Input: part model. Units: mm. Frame: model coordinates. A direction names the side the tool comes from. Give positions to 0.01 mm unless a question says otherwise; leave off trailing zeros. Loops run counter-clockwise (first coordinate to the right, second up) from the corner with the lowest first, then second, coordinate; pieces in that order, holes last. Notation, with made-up numbers: (54, -26.5) - (79, -26.5) arc R12 ccw to (79, -12.5) - close; hole circle Ø9 at (54.5, -18.5). An arc over 180 degrees is marked (long way). One line per item, written item: value.
from build123d import *

# Parameters (mm, degrees)
BOSS_EXTRUDE1_DEPTH = 12.7
SKETCH2_R           = 2.413
CUT_EXTRUDE1_DEPTH  = 55.064572735


with BuildPart() as part:
    # Sketch1 → Boss-Extrude1 (new body)
    with BuildSketch(Plane.XY):
        Polygon((0, 0), (0, 38.1), (1.905, 38.1), (1.905, 1.905), (38.1, 1.905), (38.1, 0), align=None)
    extrude(amount=BOSS_EXTRUDE1_DEPTH)

    # Sketch2 → Cut-Extrude1 (cut, through all)
    with BuildSketch(Plane(origin=(1.905, 0, 0), x_dir=(0, 0, -1), z_dir=(1, 0, 0))):
        with Locations(Location((-6.35, 30.734, 0), (0, 0, 90))):
            Circle(SKETCH2_R)
        with Locations(Location((-6.35, 12.954, 0), (0, 0, 90))):
            Circle(SKETCH2_R)
    cut_extrude1 = extrude(amount=-CUT_EXTRUDE1_DEPTH, mode=Mode.SUBTRACT)

    # Mirror1: Cut-Extrude1 across plane
    add(cut_extrude1.mirror(Plane(origin=(0, 0, 0), x_dir=(0, 0, 1), z_dir=(-0.7071067811865471, 0.7071067811865479, 0))), mode=Mode.SUBTRACT)


solid = part.part
Item 1: Draft query along X for faces 1 (the face through (38.1, 1, 6)), 2 (the face through (33.036, 0.966, 7.075)), 3 (the face through (1, 38.1, 6)). Return one class per face: pulls with the +X half, pulls with the -X half, needs draft (parallel to the pull), parting line crosses it, or undercut.
Verdict:
face 1: pulls with the +X half
face 2: undercut
face 3: needs draft
Item 2: Section B-B, the plane x = 29.5. Output: boundary loops of the cut face in (y, z) (3 decimals).
Verdict:
outline: (0, 0) - (1.905, 0) - (1.905, 4.276) - (0, 4.276) - close; (0, 8.424) - (1.905, 8.424) - (1.905, 12.7) - (0, 12.7) - close
Item 3: Access query for faces 4 (the face through (11, 1, 0)), 5 (the face through (1.905, 20, 6)). Directions: +Z, -Z, +X, -X, +Y, -Y. A direction counts if a zero-diameter tool reaches every point of the face in a straight line with its end or side. Return the directions, or none.
Verdict:
face 4: -Z, +X, -X, +Y, -Y
face 5: +Z, -Z, +X, +Y
Item 4: Section C-C, the plane y = 30.5. Output: boundary loops of the cut face in (x, z) (3 decimals), and give its area (3 significant figures).
Verdict:
outline: (0, 0) - (1.905, 0) - (1.905, 3.948) - (0, 3.948) - close; (0, 8.752) - (1.905, 8.752) - (1.905, 12.7) - (0, 12.7) - close
area: 15.0 mm^2
Item 5: Section D-D, the plane z = 10.25. Output: boundary loops of the cut face in (x, y) (3 decimals), and give its area (3 significant figures).
Verdict:
outline: (0, 0) - (38.1, 0) - (38.1, 1.905) - (1.905, 1.905) - (1.905, 38.1) - (0, 38.1) - close
area: 142 mm^2
Item 6: Section A-A, the plane z = 6.35. Output: boundary loops of the cut face in (x, y) (3 decimals).
Verdict:
outline: (0, 0) - (10.541, 0) - (10.541, 1.905) - (1.905, 1.905) - (1.905, 10.541) - (0, 10.541) - close; (0, 15.367) - (1.905, 15.367) - (1.905, 28.321) - (0, 28.321) - close; (0, 33.147) - (1.905, 33.147) - (1.905, 38.1) - (0, 38.1) - close; (15.367, 0) - (28.321, 0) - (28.321, 1.905) - (15.367, 1.905) - close; (33.147, 0) - (38.1, 0) - (38.1, 1.905) - (33.147, 1.905) - close
Item 7: Pin query (flat end, axial travel): P1, Ø6.5, axis at x = 12.954, z = 6.35, coming from the +Y side (3 decimals); P2, Ø5, axis at y = 27, z = 10.5, coming from the +X side (3 decimals). Return the tip coordinate at first contact, or that it passes through.
Verdict:
P1: stops at y = 1.905
P2: stops at x = 1.905
Item 8: Material intervals for L1, parallel to X at y = 1.2, z = 6.35; L2, parallel to X at y = 19, z = 9 (3 decimals), sorted ascending.
Verdict:
L1: x = 0 to 10.54, 15.37 to 28.32, 33.15 to 38.1
L2: x = 0 to 1.905
